Verification items for this drawing (mm, ordinates from the low corner). Round coordinates to 2 decimals unless told otherwise and drop trailing zeros. Write each loop counter-clockwise with the first axis right and the second up, starting at its lowest first coordinate (ties: lowest second). Pieces come first, ordered by that corner, then holes. Notation, with made-up numbers: M 76,77 L 80,77 A8 cw 80,90 Z; hole C 66,-37.75 d6. An arc over 180 degrees is marked long. One line per question, with ' | ' between items. Start each with the question number.
Q1. Cross-section at A-A (z = 38.5). Record the boundary of the cut face in (x, y), then the cut area to 3 significant figures.
Q2. Gauge pin test, flat ends, axial feed: pin 1 (1.6 mm diameter, centred on y = 0.5, z = 11.5, fed in from +X); pin 2 (1.2 mm diameter, centred on x = 9.5, y = 0.5, fed in from +Z); pin 3 (1 mm diameter, centred on y = 4, z = 37.5, fed in from -X); pin 4 (3.5 mm diameter, centred on x = 7, z = 74, fed in from -Y). Record the tip position at first contact, or that the pin passes through.
Q3. Thickness scan on line 1 along X through (y, z) = (1.25, 74); line 2 along X through (y, z) = (1.25, 73); line 3 along Z through (x, y) = (7, 0.4). Record the ranges inside material, lowest first. Write a range as from..to.
Q4. Cross-section at C-C (y = 2.75). Record the boundary of the cut face in (x, z), then the cut area to 3 significant figures.
Q5. Cross-section at B-B (x = 60). Record the boundary of the cut face in (y, z), then the cut area to 3 significant figures.
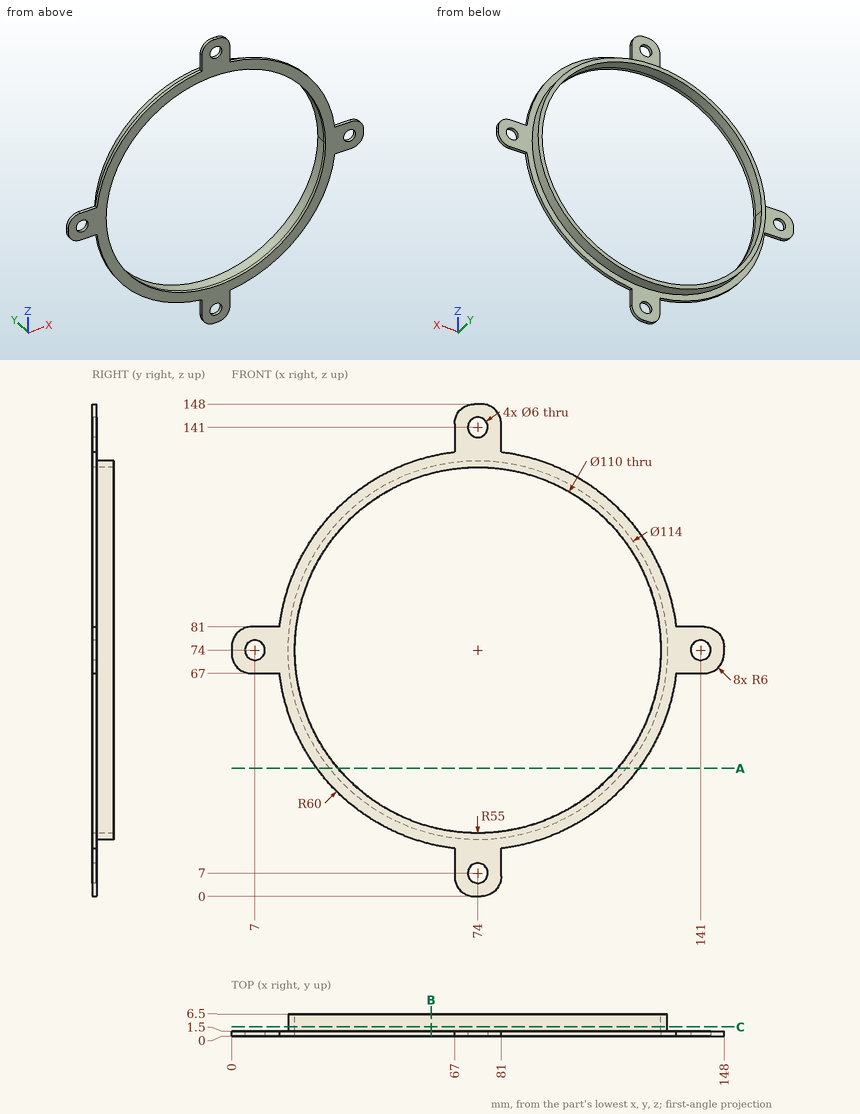
Determined:
1) outline: M 25.63,0 L 31.99,0 L 31.99,6.5 L 29.4,6.5 L 29.4,1.5 L 25.63,1.5 Z; M 116.01,0 L 122.37,0 L 122.37,1.5 L 118.6,1.5 L 118.6,6.5 L 116.01,6.5 Z | area: 45.0 mm²
2) pin 1: stops at x = 81 | pin 2: stops at z = 81 | pin 3: stops at x = 29.81 | pin 4: passes through
3) line 1: x = 0..4, 10..19, 129..138, 144..148 | line 2: x = 0..4.17, 9.83..19.01, 128.99..138.17, 143.83..148 | line 3: z = 67..71, 77..81
4) outline: C 74,74 d114; hole C 74,74 d110 | area: 704 mm²
5) outline: M 0,15.66 L 1.5,15.66 L 1.5,18.75 L 6.5,18.75 L 6.5,20.81 L 0,20.81 Z; M 0,127.19 L 6.5,127.19 L 6.5,129.25 L 1.5,129.25 L 1.5,132.34 L 0,132.34 Z | area: 36.1 mm²
